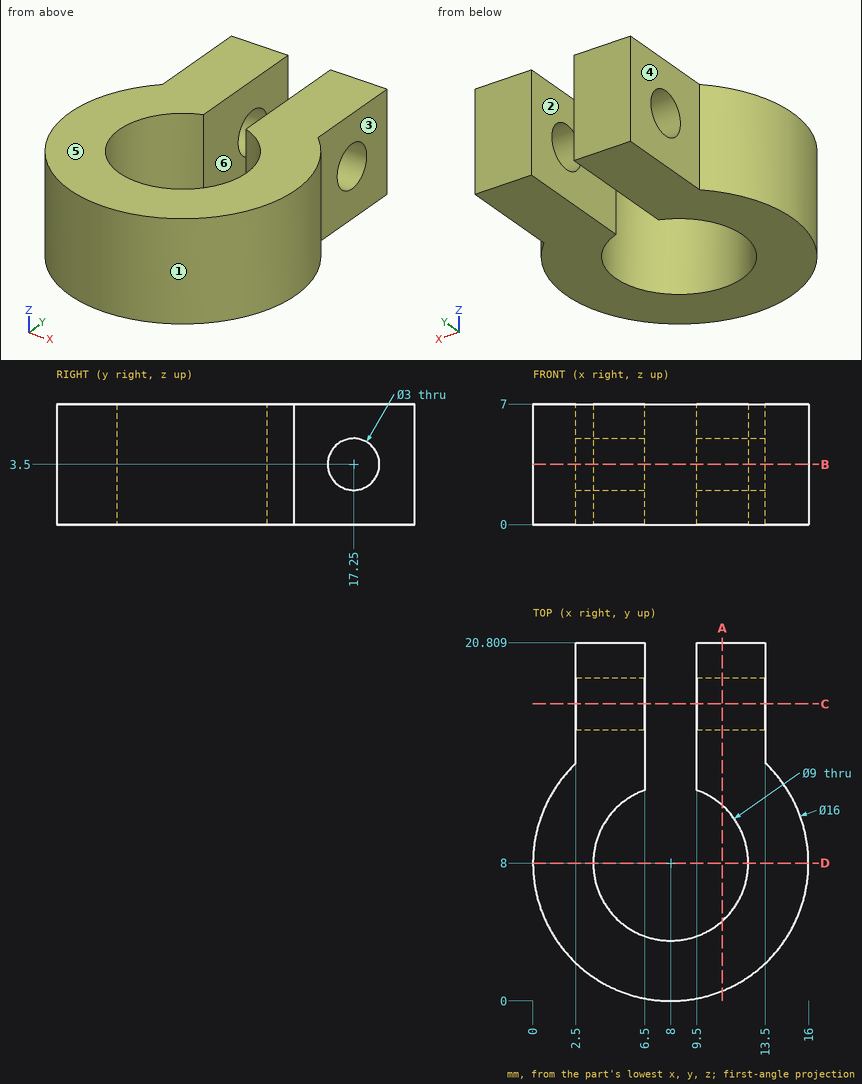
Verification items for this drawing (mm, ordinates from the low corner). A direction names the side the tool comes from. Coordinates: 2 decimals unless noted, no trailing zeros. Order: outer loops, then holes, each group sorted by start corner. A loop starts at its lowest first (then second) coordinate and runs counter-clockwise, first axis right, second up. Notation, with made-up numbers: (75, 18.25) - (97, 18.25) arc R33 cw to (97, 50.25) - close; hole circle Ø8 at (72.5, 52). An arc over 180 degrees is marked (long way). Answer as a JSON object with one key per item and string values. Group by question number.
Item 1: Sectioned sample at A-A, the plane x = 11. Give the number of separate pieces and of enclosed holes in the cut face.
Item 2: Sectioned sample at C-C, the plane y = 17.25. Record the cut outline in (x, z).
Item 3: Tool access check on the marked faces 1, 2 and 3. Record the directions out of +Z, -Z, +X, -X, +Y, -Y that give a thin tool (end or side, any length) a straight path to the whole face; none if there is none.
Item 4: Scan lines: probe 1 along X at (y, z) = (19, 3.5); probe 2 along X at (y, z) = (8, 4.25); probe 3 along Z at (x, y) = (11.5, 17.25). Record each from-to range of solid material in increasing order.
Item 5: Sectioned sample at B-B, the plane z = 3.5. Record the cut outline in (x, y).
Item 6: Sectioned sample at D-D, the plane y = 8. Record the cut outline in (x, z).
Item 7: Draft check along X on the marked faces 4, 5 and 6. Enter one of: +X half, -X half, draft (parallel to the pull), parting line (faces both ways), or undercut.
Item 8: Depth check by flat-ended pin: pin 1 Ø3.5 at (y, z) = (18.5, 2.5) entering from -X; pin 2 Ø2 at (x, z) = (13, 2) entering from -Y; pin 3 Ø3 at (y, z) = (5.5, 1.5) entering from +X. Enter the tip coordinate at first touch or a pass-through.
Resolved:
{
 "1": {"separate pieces": "2", "enclosed holes": "1"},
 "2": {"outline": "(2.5, 0) - (6.5, 0) - (6.5, 2) - (2.5, 2) - close; (2.5, 5) - (6.5, 5) - (6.5, 7) - (2.5, 7) - close; (9.5, 0) - (13.5, 0) - (13.5, 2) - (9.5, 2) - close; (9.5, 5) - (13.5, 5) - (13.5, 7) - (9.5, 7) - close"},
 "3": {"face 1": "+Z, -Z", "face 2": "+Z, -Z, +Y", "face 3": "+Z, -Z, +X, +Y"},
 "4": {"probe 1": "2.5 to 6.5, 9.5 to 13.5", "probe 2": "0 to 3.5, 12.5 to 16", "probe 3": "0 to 2, 5 to 7"},
 "5": {"outline": "(2.5, 13.81) arc R8 ccw (long way) to (13.5, 13.81) - (13.5, 15.75) - (9.5, 15.75) - (9.5, 12.24) arc R4.5 cw (long way) to (6.5, 12.24) - (6.5, 15.75) - (2.5, 15.75) - close; (2.5, 18.75) - (6.5, 18.75) - (6.5, 20.81) - (2.5, 20.81) - close; (9.5, 18.75) - (13.5, 18.75) - (13.5, 20.81) - (9.5, 20.81) - close"},
 "6": {"outline": "(0, 0) - (3.5, 0) - (3.5, 7) - (0, 7) - close; (12.5, 0) - (16, 0) - (16, 7) - (12.5, 7) - close"},
 "7": {"face 4": "-X half", "face 5": "draft", "face 6": "undercut"},
 "8": {"pin 1": "x = 2.5", "pin 2": "y = 1.07", "pin 3": "x = 15.94"}
}
